```python
from build123d import *

# Parameters (mm, degrees)
F0_R        = 2.5
F0_W        = 20
F0_H        = 20
F0_W_2      = 15.5
F0_H_2      = 15.5
F1_DEPTH    = 25
F2_START    = -7
F2_DEPTH    = 11
F3_R        = 1.5
F4_DEPTH    = 25
F5_T1_DEPTH = 35.2867319519
F5_T3_DEPTH = 34.7792924718


# Not quite as in the source:
# - a fillet or chamfer that OpenCascade refuses, or shapes differently, is made with other operations: its cross-section is extruded or revolved along the edge and cut away or added


with BuildPart() as f1:
    # F0 (on Right) → F1 (new body)
    with BuildSketch(Plane.YZ):
        Polygon((-55.5157013459, 38.3205534184), (-58.0598865449, 29.9461055547), (-38.0598865449, 29.9461055547), (-38.0598865449, 9.9461055547), (-36.6123928978, 37.3210094949), align=None)
        with BuildLine():
            ThreePointArc((-35.8098865449, 52.6961055547), (-42.207857033, 60.1146991515), (-50.4860281329, 54.8762413095))
            ThreePointArc((-50.4860281329, 54.8762413095), (-44.6074616185, 45.3092050593), (-35.8203493916, 52.3000838016))
            ThreePointArc((-35.8203493916, 52.3000838016), (-35.8125027129, 52.4980255834), (-35.8098865449, 52.6961055547))
        make_face()
        with Locations((-43.3098865449, 52.6961055547)):
            Circle(F0_R, mode=Mode.SUBTRACT)
        with Locations((-48.0598865449, 19.9461055547)):
            Rectangle(F0_W, F0_H)
        with Locations((-48.0598865449, 19.9461055547)):
            Rectangle(F0_W_2, F0_H_2, mode=Mode.SUBTRACT)
        with BuildLine():
            Line((-50.4860281329, 54.8762413095), (-55.5157013459, 38.3205534184))
            Line((-55.5157013459, 38.3205534184), (-36.6123928978, 37.3210094949))
            Line((-36.6123928978, 37.3210094949), (-35.8203493916, 52.3000838016))
            ThreePointArc((-35.8203493916, 52.3000838016), (-44.6074616185, 45.3092050593), (-50.4860281329, 54.8762413095))
        make_face()
    extrude(amount=-F1_DEPTH)

    # F0 (on Right) → F2 (cut)
    with BuildSketch(Plane.YZ.offset(F2_START)):
        with BuildLine():
            Line((-50.4860281329, 54.8762413095), (-55.5157013459, 38.3205534184))
            Line((-55.5157013459, 38.3205534184), (-36.6123928978, 37.3210094949))
            Line((-36.6123928978, 37.3210094949), (-35.8203493916, 52.3000838016))
            ThreePointArc((-35.8203493916, 52.3000838016), (-44.6074616185, 45.3092050593), (-50.4860281329, 54.8762413095))
        make_face()
        with BuildLine():
            ThreePointArc((-35.8098865449, 52.6961055547), (-42.207857033, 60.1146991515), (-50.4860281329, 54.8762413095))
            ThreePointArc((-50.4860281329, 54.8762413095), (-44.6074616185, 45.3092050593), (-35.8203493916, 52.3000838016))
            ThreePointArc((-35.8203493916, 52.3000838016), (-35.8125027129, 52.4980255834), (-35.8098865449, 52.6961055547))
        make_face()
        with Locations((-43.3098865449, 52.6961055547)):
            Circle(F0_R, mode=Mode.SUBTRACT)
    extrude(amount=-F2_DEPTH, mode=Mode.SUBTRACT)

    # F3 (on face) → F4 (cut)
    with BuildSketch(Plane.XZ.offset(58.0598865449)):
        with Locations((-12.5, 19.9461055547)):
            Circle(F3_R)
    extrude(amount=-F4_DEPTH, mode=Mode.SUBTRACT)

    # F5: chamfer of 2 on 2 edges, made by hand

    # F5_s2 → F5_t1 (cut)
    with BuildSketch(Plane.YZ.offset(-30.1433659759)):
        Polygon((-56.0598865449, 9.9461055547), (-58.0598865449, 11.9461055547), (-58.0598865449, 9.9461055547), align=None)
    extrude(amount=F5_T1_DEPTH, mode=Mode.SUBTRACT)

    # F5_s4 → F5_t3 (cut)
    with BuildSketch(Plane.YZ.offset(-29.8896462359)):
        Polygon((-37.959717296, 11.8404997539), (-39.9569272035, 9.9461055547), (-38.0598865449, 9.9461055547), align=None)
    extrude(amount=F5_T3_DEPTH, mode=Mode.SUBTRACT)


solid = f1.part
```
Design review of the part built by this model. Coordinates are the model's own, in mm. A direction names the side the tool comes from. Round coordinates to 2 decimals unless told otherwise and drop trailing zeros. Write each loop counter-clockwise with the first axis right and the second up, starting at its lowest first coordinate (ties: lowest second). Pieces come first, ordered by that corner, then holes. Notation, with made-up numbers: (85, -9) -> (121, -9) arc R15 cw to (121, 7) -> close; hole circle Ø2 at (-4.5, 86.5). An arc over 180 degrees is marked (long way). Write item = value, one per line. Start each with the question number.
1) Take a section at C-C, the plane x = -9. State the section outline as (y, z) points.
2) Tool access review of faces 1 (the face through (0, -45, 41)), 2 (the face through (-12, -48, 27.696)), 3 (the face through (-12.423, -46.196, 37.828)): name each direction out of +Z, -Z, +X, -X, +Y, -Y from which nothing blocks a thin tool from reaching the whole face with its end or side.
3) Mouldability with a two-part tool opening along Z and no side actions: class faces 4 (the face through (-12.68, -38.94, 10.91)), 5 (the face through (-12, -55.81, 22)), 6 (the face through (-7, -44, 46)) as +Z half, -Z half, draft (parallel to the pull), parting line (faces both ways), or undercut.
4) Wall thickness on probe 1 along X at (y, z) = (-40, 48); probe 2 along Z at (x, y) = (-16.5, -54.5); probe 3 along Y at (x, z) = (-7.25, 21.5): over which ranges is each line inside the solid? List them lowest first. Write a range as from..to.
5) Clearance check with flat-ended pins moving along their axes: pin 1 (5 mm diameter, centred on x = -13, z = 21, fed in from +Y); pin 2 (2 mm diameter, centred on x = -12.5, z = 37, fed in from -Y); pin 3 (2.5 mm diameter, centred on x = -12.5, z = 19.95, fed in from +Y); pin 4 (4 mm diameter, centred on x = -21, y = -45.5, fed in from +Z). State where each tip first meets the part, or that it passes through.
6) Take a section at A-A, the plane x = -22. State the section outline as (y, z) points, plus the area to 3 significant figures.
7) Take a section at B-B, the plane y = -54. State the section outline as (x, z) points.
8) Take a section at D-D, the plane x = -12.5. State the section outline as (y, z) points.
Results list:
q1.outline = (-58.06, 11.95) -> (-56.06, 9.95) -> (-39.96, 9.95) -> (-37.96, 11.84) -> (-36.61, 37.32) -> (-55.52, 38.32) -> (-58.06, 29.95) -> close; hole (-55.81, 12.2) -> (-40.31, 12.2) -> (-40.31, 27.7) -> (-55.81, 27.7) -> close
q2.face_1 = +Z, -Z, +X, +Y, -Y
q2.face_2 = +X, -X
q2.face_3 = +Z, +Y
q3.face_4 = -Z half
q3.face_5 = undercut
q3.face_6 = draft
q4.probe_1 = -25..-18, -7..0
q4.probe_2 = 9.95..12.2, 27.7..38.27
q4.probe_3 = -58.06..-55.81, -40.31..-37.45
q5.pin_1 = -37.34
q5.pin_2 = -56.22
q5.pin_3 = through
q5.pin_4 = 60.19
q6.outline = (-58.06, 11.95) -> (-56.06, 9.95) -> (-39.96, 9.95) -> (-37.96, 11.84) -> (-35.82, 52.3) arc R7.5 ccw to (-50.49, 54.88) -> (-58.06, 29.95) -> close; hole (-55.81, 12.2) -> (-40.31, 12.2) -> (-40.31, 27.7) -> (-55.81, 27.7) -> close; hole circle Ø5 at (-43.31, 52.7)
q6.area = 650 mm²
q7.outline = (-25, 9.95) -> (0, 9.95) -> (0, 12.2) -> (-25, 12.2) -> close; (-25, 27.7) -> (0, 27.7) -> (0, 43.31) -> (-7, 43.31) -> (-7, 38.24) -> (-18, 38.24) -> (-18, 43.31) -> (-25, 43.31) -> close
q8.outline = (-58.06, 11.95) -> (-56.06, 9.95) -> (-39.96, 9.95) -> (-37.96, 11.84) -> (-37.61, 18.45) -> (-40.31, 18.45) -> (-40.31, 12.2) -> (-55.81, 12.2) -> (-55.81, 18.45) -> (-58.06, 18.45) -> close; (-58.06, 21.45) -> (-55.81, 21.45) -> (-55.81, 27.7) -> (-40.31, 27.7) -> (-40.31, 21.45) -> (-37.45, 21.45) -> (-36.61, 37.32) -> (-55.52, 38.32) -> (-58.06, 29.95) -> close
